```python
from build123d import *

# Parameters (mm, degrees)
SMUSSO1_SIZE             = 1
SCHIZZO2_R               = 6
TAGLIO_ESTRUSIONE1_DEPTH = 38.259227045
SCHIZZO3_R               = 1.65
TAGLIO_ESTRUSIONE2_DEPTH = 32.75787304


with BuildPart() as part:
    # Schizzo1 → Rivoluzione1 (revolve)
    with BuildSketch(Plane.XY, mode=Mode.PRIVATE) as rivoluzione1_sk:
        Polygon((0, 11.25), (13.45, 11.25), (13.45, 3.25), (21, 3.25), (21, 1.5), (18.5, 1.5), (18.5, -9.5), (21, -9.5), (21, -11.25), (0, -11.25), align=None)
    revolve(rivoluzione1_sk.sketch.rotate(Axis((0, -12.375, 0), (0, 1, 0)), 90), axis=Axis((0, -12.375, 0), (0, 1, 0)))

    # Smusso1
    smusso1_edges = [part.edges().sort_by_distance(p)[0] for p in [
        (0, 11.25, 13.45),
    ]]
    chamfer(smusso1_edges, length=SMUSSO1_SIZE)

    # Schizzo2 → Taglio-Estrusione1 (cut, through all)
    with BuildSketch(Plane(origin=(0, 11.25, 0), x_dir=(1, 0, 0), z_dir=(0, 1, 0))):
        with Locations(Location((0, 0, 0), (0, 0, 270))):
            Circle(SCHIZZO2_R)
    extrude(amount=-TAGLIO_ESTRUSIONE1_DEPTH, mode=Mode.SUBTRACT)

    # Schizzo3 → Taglio-Estrusione2 (cut, through all)
    with BuildSketch(Plane.XY):
        with Locations((0, 6.75)):
            Circle(SCHIZZO3_R)
    extrude(amount=-TAGLIO_ESTRUSIONE2_DEPTH, mode=Mode.SUBTRACT)


solid = part.part
```
Design review of the part built by this model. Coordinates are the model's own, in mm. A direction names the side the tool comes from. Give positions to 0.01 mm unless a question says otherwise; leave off trailing zeros. Order: outer loops, then holes, each group sorted by start corner. A loop starts at its lowest first (then second) coordinate and runs counter-clockwise, first axis right, second up. Notation, with made-up numbers: (27.5, 77.5) - (48.5, 77.5) arc R19 ccw to (48.5, 85.5) - close; hole circle Ø7 at (-34, 9.5). An arc over 180 degrees is marked (long way). Use a Markdown table: item, result. Add a question column.
(1) Clearance check with flat-ended pins moving along their axes: P1, Ø4.5, axis at x = 0, y = 6.75, coming from the -Z side; P2, Ø10, axis at y = -8, z = -9, coming from the +X side; P3, Ø3, axis at x = -13.5, y = 4, coming from the -Z side. State where each tip first meets the part, or that it passes through.
(2) Add section C-C on y = -8.75. Give the boundary of the cut face in (x, z), then the cut area to 3 significant figures.
(3) Add section B-B on x = 0. Give the boundary of the cut face in (y, z), then the cut area to 3 significant figures.
(4) Mouldability with a two-part tool opening along Y and no side actions: class faces 1 (the face through (4.4, -11.25, -4.4)), 2 (the face through (19, 1.5, 0)), 3 (the face through (-6.31, 2.36, -20.03)) as +Y half, -Y half, draft (parallel to the pull), parting line (faces both ways), or undercut.
(5) Add section D-D on x = -16.5. Give the boundary of the cut face in (y, z), then the cut area to 3 significant figures.
(6) Add section A-A on z = 0. Give the boundary of the cut face in (x, y), then the cut area to 3 significant figures.
(7) Machinability: for faces 4 (the face through (14, 3.25, 0)), 5 (the face through (-6.31, -10.39, -20.03)), 6 (the face through (-0.36, 5.14, -9.55)), 7 (the face through (-6, 11.25, 3)), 8 (the face through (19, -9.5, 0)), which of the approach directions +Z, -Z, +X, -X, +Y, -Y give a long, thin tool a straight path to every point of the face, cutting with its end or side? Answer none if there is none.
(8) Wall thickness on probe 1 along Y at (x, z) = (17.5, 8.5); probe 2 along X at (y, z) = (-3.25, 0); probe 3 along Y at (x, z) = (11, 11.5): over which ranges is each line inside the solid? List them lowest first. Write a range as [from, to].
Report:
| question | item | result |
|---|---|---|
| 1 | P1 | stops at z = -13.45 |
| 1 | P2 | stops at x = 20.57 |
| 1 | P3 | stops at z = -17.09 |
| 2 | outline | circle Ø37 at (0, 0); hole circle Ø12 at (0, 0) |
| 2 | area | 962 mm² |
| 3 | outline | (-11.25, -21) - (-9.5, -21) - (-9.5, -18.5) - (1.5, -18.5) - (1.5, -21) - (3.25, -21) - (3.25, -13.45) - (5.1, -13.45) - (5.1, -6) - (-11.25, -6) - close; (-11.25, 6) - (11.25, 6) - (11.25, 12.45) - (10.25, 13.45) - (3.25, 13.45) - (3.25, 21) - (1.5, 21) - (1.5, 18.5) - (-9.5, 18.5) - (-9.5, 21) - (-11.25, 21) - close; (8.4, -13.45) - (10.25, -13.45) - (11.25, -12.45) - (11.25, -6) - (8.4, -6) - close |
| 3 | area | 474 mm² |
| 4 | face 1 | -Y half |
| 4 | face 2 | undercut |
| 4 | face 3 | draft |
| 5 | outline | (-11.25, -12.99) - (-9.5, -12.99) - (-9.5, -8.37) - (1.5, -8.37) - (1.5, -12.99) - (3.25, -12.99) - (3.25, 12.99) - (1.5, 12.99) - (1.5, 8.37) - (-9.5, 8.37) - (-9.5, 12.99) - (-11.25, 12.99) - close |
| 5 | area | 275 mm² |
| 6 | outline | (-21, -11.25) - (-6, -11.25) - (-6, 11.25) - (-12.45, 11.25) - (-13.45, 10.25) - (-13.45, 3.25) - (-21, 3.25) - (-21, 1.5) - (-18.5, 1.5) - (-18.5, -9.5) - (-21, -9.5) - close; (6, -11.25) - (21, -11.25) - (21, -9.5) - (18.5, -9.5) - (18.5, 1.5) - (21, 1.5) - (21, 3.25) - (13.45, 3.25) - (13.45, 10.25) - (12.45, 11.25) - (6, 11.25) - close |
| 6 | area | 498 mm² |
| 7 | face 4 | +Y |
| 7 | face 5 | +Y, -Y |
| 7 | face 6 | -Z |
| 7 | face 7 | +Z, -Z, +X, -X, +Y |
| 7 | face 8 | none |
| 8 | probe 1 | y = [-11.25, -9.5], [1.5, 3.25] |
| 8 | probe 2 | x = [-18.5, -6], [6, 18.5] |
| 8 | probe 3 | y = [-11.25, 3.25] |
